For this review, take the finished solid that the model builds, in its own axes (mm). Face numbers are marked on the shaded views. A direction names the side the tool comes from. Round coordinates to 2 decimals unless told otherwise and drop trailing zeros. Write each loop counter-clockwise with the first axis right and the second up, starting at its lowest first coordinate (ties: lowest second). Pieces come first, ordered by that corner, then holes. Notation, with made-up numbers: (70.5, -11.75) -> (126.5, -11.75) arc R10 cw to (126.5, -0.75) -> close; hole circle Ø5 at (84, -14.5). An arc over 180 degrees is marked (long way). Answer in a Markdown table with one row per item.
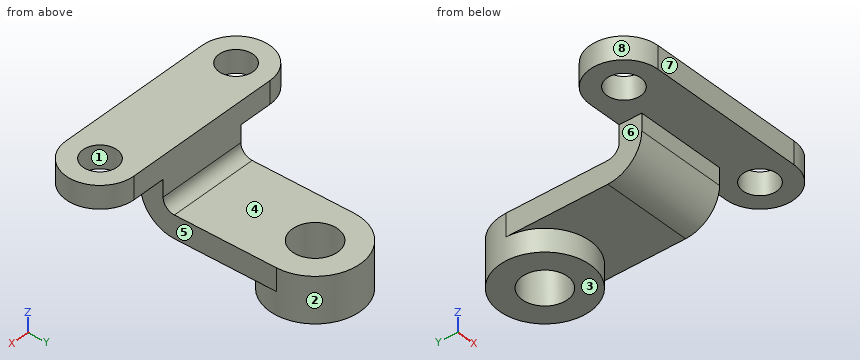
Autodesk Inventor part; units mm, degrees
ref_plane "YZ Plane" through (0, 0, 0) normal (1, 0, 0) x (0, 1, 0)
ref_plane "XZ Plane" through (0, 0, 0) normal (0, 1, 0) x (-1, 0, 0)
ref_plane "XY Plane" through (0, 0, 0) normal (0, 0, 1) x (1, 0, 0)
sketch "SLOT SK" plane through (0, 0, 0) normal (0, 0, 1) x (1, 0, 0)
  line L0 (-88.9, 0) -> (88.9, 0) construction
  line L1 (-88.9, -38.1) -> (88.9, -38.1)
  line L2 (88.9, 38.1) -> (-88.9, 38.1)
  arc A0 (-88.9, 38.1) -> (-88.9, -38.1) centre (-88.9, 0) ccw
  arc A1 (88.9, -38.1) -> (88.9, 38.1) centre (88.9, 0) ccw
  circle A2 centre (-88.9, 0) radius 19.05
  circle A3 centre (88.9, 0) radius 19.05
  point P0 (0, 0)
  point P1 (0, 0)
  dimension "d0" = 177.8
  dimension "d1" = 88.9
  dimension "d2" = 38.1
  dimension "d3" = 38.1
  dimension "d4" = 38.1
extrude "SLOT EXT" add sketch "SLOT SK" along normal blind 25.4
sketch "Sketch2" plane through (0, 0, 0) normal (1, 0, 0) x (0, 1, 0)
  line L0 (38.1, 0) -> (-38.1, 0)
  line L1 (12.7, 0) -> (38.1, 0)
  line L2 (38.1, 0) -> (38.1, -19.05)
  line L3 (50.8, -31.75) -> (165.1, -31.75)
  line L4 (165.1, -31.75) -> (165.1, -57.15)
  line L5 (165.1, -57.15) -> (50.8, -57.15)
  line L6 (12.7, -19.05) -> (12.7, 0)
  arc A0 (38.1, -19.05) -> (50.8, -31.75) centre (50.8, -19.05) ccw
  arc A1 (12.7, -19.05) -> (50.8, -57.15) centre (50.8, -19.05) ccw
  line L7 (38.1, 0) -> (38.1, 25.4)
  line L8 (38.1, 25.4) -> (-38.1, 25.4)
  point P0 (0, 0)
  dimension "d7" = 12.7
  dimension "d8" = 38.1
  dimension "d9" = 127
  dimension "d10" = 57.15
  dimension "d11" = 25.4
  dimension "d12" = 25.4
extrude "J JOINT" add sketch "Sketch2" along normal mid plane 101.6
sketch "TOP JOINT" plane through (-50.8, 50.8, -31.75) normal (0, 0, 1) x (1, 0, 0)
  line L0 (0, 114.3) -> (101.6, 114.3)
  line L1 (101.6, 0) -> (101.6, 114.3)
  circle A0 centre (50.8, 114.3) radius 50.8
  circle A1 centre (50.8, 114.3) radius 25.4
  point P0 (50.8, -50.8)
  point P1 (76.2, 114.3)
  point P2 (25.4, 114.3)
  dimension "d15" = 50.8
extrude "TOP CYLINDER" add sketch "TOP JOINT" against normal blind 50.8 contours A1 L0 A0 | L0 A0 A1
extrude "TOP HOLE" cut sketch "TOP JOINT" against normal blind 101.6 contours A1 L0 picked at (54.5078, 94.9925)
equation "\"d4\" = d3"
properties part number "ASN5-6-BK" material "Thermoplastic Resin"
1) Consider section B-B on x = 0. State the section outline as (y, z) points, then the cut area to 3 significant figures.
Solved:
| item | result |
|---|---|
| outline | (-38.1, 0) -> (12.7, 0) -> (12.7, -19.05) arc R38.1 ccw to (50.8, -57.15) -> (114.3, -57.15) -> (114.3, -82.55) -> (139.7, -82.55) -> (139.7, -31.75) -> (50.8, -31.75) arc R12.7 cw to (38.1, -19.05) -> (38.1, 25.4) -> (-38.1, 25.4) -> close; (190.5, -82.55) -> (215.9, -82.55) -> (215.9, -31.75) -> (190.5, -31.75) -> close |
| area | 7,630 mm² |
2) Clearance check with flat-ended pins moving along their axes: pin 1 Ø12 at (y, z) = (131, -30.5) entering from -X; pin 2 Ø5 at (x, y) = (37, -3.5) entering from -Z; pin 3 Ø1.5 at (x, z) = (5, 1) entering from +Y. State where each tip first meets the part, or that it passes through.
Solved:
| item | result |
|---|---|
| pin 1 | x = -50.8 |
| pin 2 | z = 0 |
| pin 3 | y = 38.1 |
3) For the marked faces 4, 5, 6, 7 and 8, list the 3-axis set-ups (+Z, -Z, +X, -X, +Y, -Y) from which the entire face can be reached by the end or side of a thin tool; tool diameter is ignored.
Solved:
| item | result |
|---|---|
| face 4 | +Z, +X, -X, +Y |
| face 5 | -Z, +X, +Y, -Y |
| face 6 | -Z, -X, +Y, -Y |
| face 7 | +Z, -Z, +X, -X, -Y |
| face 8 | +Z, -Z, -X |
4) Consider section D-D on y = 182. State the section outline as (x, z) points, then the cut area to 3 significant figures.
Solved:
| item | result |
|---|---|
| outline | (-47.91, -82.55) -> (-18.96, -82.55) -> (-18.96, -31.75) -> (-47.91, -31.75) -> close; (18.96, -82.55) -> (47.91, -82.55) -> (47.91, -31.75) -> (18.96, -31.75) -> close |
| area | 2,940 mm² |
5) Consider section C-C on z = 6. State the section outline as (x, y) points.
Solved:
| item | result |
|---|---|
| outline | (-88.9, -38.1) -> (88.9, -38.1) arc R38.1 ccw to (88.9, 38.1) -> (-88.9, 38.1) arc R38.1 ccw to start; hole circle Ø38.1 at (-88.9, 0); hole circle Ø38.1 at (88.9, 0) |
6) For line 1 (Y direction, x = -88.9, z = 12.5); line 2 (X direction, y = 165, z = -54); line 3 (Z direction, x = -1.5, y = 96), list the stretches that pass through material, from the lowest coordinate up. Write a range as [from, to].
Solved:
| item | result |
|---|---|
| line 1 | [-38.1, -19.05], [19.05, 38.1] |
| line 2 | [-50.8, -25.4], [25.4, 50.8] |
| line 3 | [-57.15, -31.75] |
7) Mouldability with a two-part tool opening along Y and no side actions: class the marked faces 1, 2 and 3 as pulls with the +Y half, pulls with the -Y half, needs draft (parallel to the pull), parting line crosses it, or undercut.
Solved:
| item | result |
|---|---|
| face 1 | undercut |
| face 2 | parting line crosses it |
| face 3 | needs draft |
8) Consider section A-A on y = 0. State the section outline as (x, z) points.
Solved:
| item | result |
|---|---|
| outline | (-127, 0) -> (-107.95, 0) -> (-107.95, 25.4) -> (-127, 25.4) -> close; (-69.85, 0) -> (69.85, 0) -> (69.85, 25.4) -> (-69.85, 25.4) -> close; (107.95, 0) -> (127, 0) -> (127, 25.4) -> (107.95, 25.4) -> close |
